Part model, mm, in its own coordinate system. Face numbers are marked on the shaded views. A direction names the side the tool comes from. Give positions to 0.01 mm unless a question says otherwise; leave off trailing zeros. Write each loop counter-clockwise with the first axis right and the second up, starting at its lowest first coordinate (ties: lowest second). Pieces come first, ordered by that corner, then holes. Notation, with made-up numbers: M -6.5,85 L 6.5,85 A32 cw 6.5,113 Z; hole C 22.25,12.25 d4. An arc over 180 degrees is marked long. Write item = value, one per line. Start each with the question number.
Autodesk Inventor part; units mm, degrees
ref_plane "작업 평면1" through (-12.5, 3.2, 3.2) normal (0, 0.7071, -0.7071) x (-1, 0, 0)
ref_plane "YZ Plane" through (0, 0, 0) normal (1, 0, 0) x (0, 1, 0)
ref_plane "XZ Plane" through (0, 0, 0) normal (0, 1, 0) x (-1, 0, 0)
sketch "스케치1" plane through (0, 0, 0) normal (1, 0, 0) x (0, 1, 0)
  line L0 (0, 10) -> (0, 30)
  line L1 (0, 30) -> (3.2, 30)
  line L2 (3.2, 30) -> (3.2, 3.2)
  line L3 (3.2, 3.2) -> (30, 3.2)
  line L4 (30, 3.2) -> (30, 0)
  line L5 (30, 0) -> (0, 0)
  line L6 (0, 0) -> (0, 10)
  dimension "d2" = 3.2
  dimension "d3" = 26.8
  dimension "d4" = 26.8
  dimension "d5" = 90
  dimension "d6" = 3.2
  dimension "d13" = 90
  dimension "d14" = 10
extrude "돌출1" add sketch "스케치1" along normal mid plane 25
sketch "스케치2" plane through (-12.5, 3.2, 30) normal (0, 1, 0) x (1, 0, 0)
  line L0 (12.5, 10) -> (12.5, 16) construction
  line L1 (16, 10) -> (16, 16)
  line L2 (9, 16) -> (9, 10)
  arc A0 (9, 10) -> (16, 10) centre (12.5, 10) ccw
  arc A1 (16, 16) -> (9, 16) centre (12.5, 16) ccw
  line L3 (0, 0) -> (25, 0)
  line L4 (0, 0) -> (0, 26.8)
  point P0 (12.5, 30)
  point P1 (12.5, 13)
  point P2 (0, 13.4)
  dimension "d10" = 6
  dimension "d11" = 7
  dimension "d12" = 10
  dimension "d15" = 12.5
extrude "돌출2" cut sketch "스케치2" against normal through all
ref_plane "작업 평면1" through (-12.5, 3.2, 3.2) normal (0, 0.7071, -0.7071) x (-1, 0, 0)
mirror "미러1" about plane through (-12.5, 3.2, 3.2) normal (0, 0.7071, -0.7071) of "돌출2"
fillet "모깎기2" radius 1 11 edges at (12.5, 16.6, 3.2) (0, 30, 3.2) (-12.5, 16.6, 3.2) (12.5, 3.2, 16.6) (0, 3.2, 30) (-12.5, 3.2, 16.6) (0, 3.2, 3.2) (12.5, 30, 1.6) (-12.5, 30, 1.6) (-12.5, 1.6, 30) (12.5, 1.6, 30)
fillet "모깎기3" radius 3.2 1 edges at (0, 0, 0)
properties part number "안쪽브라켓"
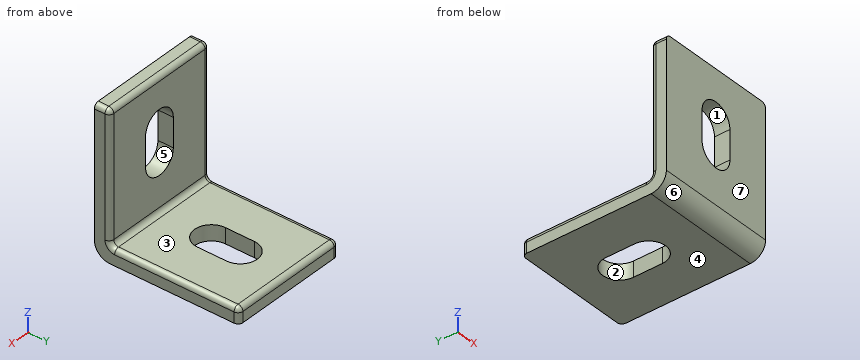
Q1. Slice it at C-C (z = 26.5). Give the cut face in (x, y).
Q2. Drop flat-ended pins along their axis: P1, Ø12, axis at x = -8, z = 20.5, coming from the +Y side; P2, Ø8, axis at x = 6.5, y = 8.5, coming from the +Z side. Give the stop position or say it passes through.
Q3. Probe line 1 along Z through (x, y) = (4, 28.5); line 2 along X through (y, z) = (21, 3). List the from-to ranges inside material, lowest first.
Q4. Slice it at B-B (x = 5.75). Give the cut face in (y, z), and give its area (3 significant figures).
Q5. Two-plate mould, pull along Z, no slides. Class the marked faces 5, 6 and 7: +Z half, -Z half, draft (parallel to the pull), parting line (faces both ways), or undercut.
Q6. Tool access for the marked faces 1, 2, 3 and 4: list every direction of +Z, -Z, +X, -X, +Y, -Y with a clear straight run to the whole face (end or side of a thin tool).
Q7. Slice it at A-A (x = 0). Give the cut face in (y, z), and give its area (3 significant figures).
Working result:
q1.outline = M -12.5,0 L 12.5,0 L 12.5,2.2 A1 ccw 11.5,3.2 L -11.5,3.2 A1 ccw -12.5,2.2 Z
q2.P1 = 3.2
q2.P2 = 3.2
q3.line_1 = 0 to 3.2
q3.line_2 = -12.1 to -3.35, 3.35 to 12.1
q4.outline = M 0,3.2 A3.2 ccw 3.2,0 L 30,0 L 30,2.2 A1 ccw 29,3.2 L 4.2,3.2 A1 cw 3.2,4.2 L 3.2,29 A1 ccw 2.2,30 L 0,30 Z
q4.area = 179 mm2
q5.face_5 = undercut
q5.face_6 = -Z half
q5.face_7 = draft
q6.face_1 = +Y, -Y
q6.face_2 = +Z, -Z
q6.face_3 = +Z, +X, -X, +Y
q6.face_4 = -Z, +X, -X, +Y, -Y
q7.outline = M 0,3.2 A3.2 ccw 3.2,0 L 10.5,0 L 10.5,3.2 L 4.2,3.2 A1 cw 3.2,4.2 L 3.2,10.5 L 0,10.5 Z; M 0,23.5 L 3.2,23.5 L 3.2,29 A1 ccw 2.2,30 L 0,30 Z; M 23.5,0 L 30,0 L 30,2.2 A1 ccw 29,3.2 L 23.5,3.2 Z
q7.area = 96.1 mm2
